```python
from build123d import *

# Parameters (mm, degrees)
SKETCH3_W           = 23
SKETCH3_H           = 7.38
BOSS_EXTRUDE1_DEPTH = 7.76
SKETCH4_R           = 3.1
CUT_EXTRUDE2_DEPTH  = 0.8
SKETCH7_R           = 3.1
CUT_EXTRUDE3_DEPTH  = 0.8
SKETCH6_R           = 2.5
CUT_EXTRUDE4_DEPTH  = 7.96
FILLET3_R           = 2
FILLET4_R           = 2
FILLET5_R           = 2
FILLET6_R           = 2
SKETCH8_W           = 3
SKETCH8_H           = 3
BOSS_EXTRUDE2_DEPTH = 6.115
SKETCH9_R           = 1.425
BOSS_EXTRUDE3_DEPTH = 25.6
SKETCH12_W          = 3
SKETCH12_H          = 3
BOSS_EXTRUDE4_DEPTH = 6.115
SKETCH13_R          = 1.425
BOSS_EXTRUDE5_DEPTH = 25.6


with BuildPart() as part:
    # Sketch3 → Boss-Extrude1 (new body)
    with BuildSketch(Plane(origin=(0, 0, 0), x_dir=(1, 0, 0), z_dir=(0, 1, 0))):
        with Locations((-11.5, 3.69)):
            Rectangle(SKETCH3_W, SKETCH3_H)
    extrude(amount=BOSS_EXTRUDE1_DEPTH)

    # Sketch4 → Cut-Extrude2 (cut)
    with BuildSketch(Plane(origin=(0, 0, 0), x_dir=(-1, 0, 0), z_dir=(0, -1, 0))):
        with Locations((19.538269405, 3.69)):
            Circle(SKETCH4_R)
        with Locations((11.538269405, 3.69)):
            Circle(SKETCH4_R)
        with Locations((3.538269405, 3.69)):
            Circle(SKETCH4_R)
    extrude(amount=-CUT_EXTRUDE2_DEPTH, mode=Mode.SUBTRACT)

    # Sketch7 → Cut-Extrude3 (cut)
    with BuildSketch(Plane(origin=(0, 7.76, 0), x_dir=(1, 0, 0), z_dir=(0, 1, 0))):
        with Locations((-19.478269405, 3.591470107)):
            Circle(SKETCH7_R)
        with Locations((-11.508269405, 3.591470107)):
            Circle(SKETCH7_R)
        with Locations((-3.538269405, 3.591470107)):
            Circle(SKETCH7_R)
    extrude(amount=-CUT_EXTRUDE3_DEPTH, mode=Mode.SUBTRACT)

    # Sketch6 → Cut-Extrude4 (cut, through all)
    with BuildSketch(Plane(origin=(0, 0.8, 0), x_dir=(-1, 0, 0), z_dir=(0, -1, 0))):
        with Locations((3.538269405, 3.591470107)):
            Circle(SKETCH6_R)
        with Locations((11.508269405, 3.591470107)):
            Circle(SKETCH6_R)
        with Locations((19.478269405, 3.591470107)):
            Circle(SKETCH6_R)
    extrude(amount=-CUT_EXTRUDE4_DEPTH, mode=Mode.SUBTRACT)

    # Fillet3
    fillet3_edges = [part.edges().sort_by_distance(p)[0] for p in [
        (0, 3.88, 0),
    ]]
    fillet(fillet3_edges, radius=FILLET3_R)

    # Fillet4
    fillet4_edges = [part.edges().sort_by_distance(p)[0] for p in [
        (-23, 3.88, 0),
    ]]
    fillet(fillet4_edges, radius=FILLET4_R)

    # Fillet5
    fillet5_edges = [part.edges().sort_by_distance(p)[0] for p in [
        (-23, 3.88, -7.38),
    ]]
    fillet(fillet5_edges, radius=FILLET5_R)

    # Fillet6
    fillet6_edges = [part.edges().sort_by_distance(p)[0] for p in [
        (0, 3.88, -7.38),
    ]]
    fillet(fillet6_edges, radius=FILLET6_R)

    # Sketch8 → Boss-Extrude2 (add)
    with BuildSketch(Plane(origin=(0, 0, -7.38), x_dir=(-1, 0, 0), z_dir=(0, 0, -1))):
        with Locations((15.65, 6.200251459)):
            Rectangle(SKETCH8_W, SKETCH8_H)
    extrude(amount=BOSS_EXTRUDE2_DEPTH)

    # Sketch9 → Boss-Extrude3 (add)
    with BuildSketch(Plane(origin=(0, 7.700251459, 0), x_dir=(1, 0, 0), z_dir=(0, 1, 0))):
        with Locations((-15.65, 12.081963091)):
            Circle(SKETCH9_R)
    extrude(amount=BOSS_EXTRUDE3_DEPTH)

    # Sketch12 → Boss-Extrude4 (add)
    with BuildSketch(Plane.XY):
        with Locations((-15.65, 5.962808026)):
            Rectangle(SKETCH12_W, SKETCH12_H)
    extrude(amount=BOSS_EXTRUDE4_DEPTH)

    # Sketch13 → Boss-Extrude5 (add)
    with BuildSketch(Plane(origin=(0, 7.462808026, 0), x_dir=(1, 0, 0), z_dir=(0, 1, 0))):
        with Locations((-15.65, -4.763284268)):
            Circle(SKETCH13_R)
    extrude(amount=BOSS_EXTRUDE5_DEPTH)


solid = part.part
```
CAD build for the part. Positions are in the model's coordinates, mm. A direction names the side the tool comes from. Round coordinates to 2 decimals unless told otherwise and drop trailing zeros. Write each loop counter-clockwise with the first axis right and the second up, starting at its lowest first coordinate (ties: lowest second). Pieces come first, ordered by that corner, then holes. Notation, with made-up numbers: (80.25, 16) -> (91.25, 16) arc R23 cw to (91.25, 28) -> close; hole circle Ø6 at (-33.75, 47.25). An arc over 180 degrees is marked (long way). Answer in a Markdown table with one row per item. Add a question column.
Item 1: Which spindle directions (+Z, -Z, +X, -X, +Y, -Y) get a long thin tool onto all of the face, cutting with end or side? Do faces 4 (the face through (-14.15, 6, 3)), 5 (the face through (-15.8, 20.3, -13.5)), 6 (the face through (-16.44, 0.39, -3.83)), 7 (the face through (-14.15, 6, -10)). Say none if no direction does.
Item 2: Saw through at B-B, the plane y = 4. Write the cut outline in (x, z).
Item 3: Saw through at A-A, the plane x = -21.5. Write the cut outline in (y, z).
Item 4: Saw through at C-C, the plane z = 0.75. Write the cut outline in (x, y).
Item 5: Drop flat-ended pins along their axis: pin 1 Ø5 at (x, z) = (-19, -7) entering from +Y; pin 2 Ø3 at (x, z) = (-16.5, 4.5) entering from +Y; pin 3 Ø1.5 at (x, z) = (-15.5, 2) entering from -Y; pin 4 Ø10 at (x, y) = (-7.5, 28.5) entering from +Z. Give the stop position or say it passes through.
Item 6: Saw through at D-D, the plane x = -7.5. Write the cut outline in (y, z).
Item 7: Drill centre lines: line 1 (Y direction, x = -13, z = -0.5); line 2 (Z direction, x = -15.25, y = 3.5); line 3 (Y direction, x = -16, z = 5.25). Where is each one in solid material? Low to high. Write a range as from..to.
Item 8: Mould opens along Z. For faces 1 (the face through (-0.6, 3.93, -0.57)), 2 (the face through (-16.52, 7.37, -4.52)), 3 (the face through (-12, 0, -7)) say: pulls with the +Z half, pulls with the -Z half, needs draft (parallel to the pull), parting line crosses it, or undercut.
Findings below:
| question | item | result |
|---|---|---|
| 1 | face 4 | +Z, +X, +Y, -Y |
| 1 | face 5 | +Y |
| 1 | face 6 | -Y |
| 1 | face 7 | -Z, +X, +Y, -Y |
| 2 | outline | (-23, -5.38) arc R2 ccw to (-21, -7.38) -> (-2, -7.38) arc R2 ccw to (0, -5.38) -> (0, -2) arc R2 ccw to (-2, 0) -> (-21, 0) arc R2 ccw to (-23, -2) -> close; hole circle Ø5 at (-19.48, -3.59); hole circle Ø5 at (-11.51, -3.59); hole circle Ø5 at (-3.54, -3.59) |
| 3 | outline | (0, -7.32) -> (7.76, -7.32) -> (7.76, -5.94) -> (6.96, -5.94) -> (6.96, -5.06) -> (0.8, -5.06) -> (0.8, -6.09) -> (0, -6.09) -> close; (0, -1.29) -> (0.8, -1.29) -> (0.8, -2.12) -> (6.96, -2.12) -> (6.96, -1.24) -> (7.76, -1.24) -> (7.76, -0.06) -> (0, -0.06) -> close |
| 4 | outline | (-17.15, 4.46) -> (-14.15, 4.46) -> (-14.15, 7.46) -> (-17.15, 7.46) -> close |
| 5 | pin 1 | stops at y = 7.76 |
| 5 | pin 2 | stops at y = 33.06 |
| 5 | pin 3 | stops at y = 4.46 |
| 5 | pin 4 | passes through |
| 6 | outline | (0, -7.38) -> (7.76, -7.38) -> (7.76, 0) -> (0, 0) -> close |
| 7 | line 1 | y = 0..7.76 |
| 7 | line 2 | z = -7.38..0 |
| 7 | line 3 | y = 4.46..33.06 |
| 8 | face 1 | pulls with the +Z half |
| 8 | face 2 | undercut |
| 8 | face 3 | needs draft |
